```python
from build123d import *

# Parameters (mm, degrees)
SKETCH1_W               = 56
SKETCH1_H               = 32
BOSS_EXTRUDE1_DEPTH     = 2
SKETCH2_R               = 1.75
CUT_EXTRUDE1_DEPTH      = 33.310988843
MIRROR2_COPY_1_SKETCH_R = 1.75
MIRROR2_COPY_1_DEPTH    = 33.310988843
SKETCH4_W               = 14.25
SKETCH4_H               = 7.5
CUT_EXTRUDE2_DEPTH      = 33.310988843
MIRROR4_COPY_1_SKETCH_W = 14.25
MIRROR4_COPY_1_SKETCH_H = 7.5
MIRROR4_COPY_1_DEPTH    = 33.310988843
SKETCH5_W               = 56
SKETCH5_H               = 32
SKETCH5_W_2             = 50
SKETCH5_H_2             = 26
BOSS_EXTRUDE2_DEPTH     = 4.65
SKETCH6_W               = 51
SKETCH6_H               = 27
SKETCH6_W_2             = 50
SKETCH6_H_2             = 26
BOSS_EXTRUDE3_DEPTH     = 1
FILLET1_R               = 1


with BuildPart() as part:
    # Sketch1 → Boss-Extrude1 (new body)
    with BuildSketch(Plane(origin=(0, 0, 0), x_dir=(1, 0, 0), z_dir=(0, 1, 0))):
        Rectangle(SKETCH1_W, SKETCH1_H)
    extrude(amount=BOSS_EXTRUDE1_DEPTH)

    # Sketch2 → Cut-Extrude1 (cut, through all)
    with BuildSketch(Plane(origin=(0, 0, 0), x_dir=(1, 0, 0), z_dir=(0, 1, 0))):
        with Locations(Location((20, 6.5, 0), (0, 0, 270))):
            Circle(SKETCH2_R)
    cut_extrude1 = extrude(amount=CUT_EXTRUDE1_DEPTH, mode=Mode.SUBTRACT)

    # Mirror1: Cut-Extrude1 across plane
    add(cut_extrude1.mirror(Plane.XY), mode=Mode.SUBTRACT)

    # Mirror2: Cut-Extrude1 across plane
    add(cut_extrude1.mirror(Plane(origin=(0, 0, 0), x_dir=(0, 0, 1), z_dir=(1, 0, 0))), mode=Mode.SUBTRACT)

    # Mirror2 copy 1 sketch → Mirror2 copy 1 (cut, through all)
    with BuildSketch(Plane(origin=(0, 0, 0), x_dir=(-1, 0, 0), z_dir=(0, 1, 0))):
        with Locations(Location((20, 6.5, 0), (0, 0, 270))):
            Circle(MIRROR2_COPY_1_SKETCH_R)
    extrude(amount=MIRROR2_COPY_1_DEPTH, mode=Mode.SUBTRACT)

    # Sketch4 → Cut-Extrude2 (cut, through all)
    with BuildSketch(Plane(origin=(0, 0, 0), x_dir=(1, 0, 0), z_dir=(0, 1, 0))):
        with Locations((8.46, 6.875)):
            Rectangle(SKETCH4_W, SKETCH4_H)
    cut_extrude2 = extrude(amount=CUT_EXTRUDE2_DEPTH, mode=Mode.SUBTRACT)

    # Mirror3: Cut-Extrude2 across plane
    add(cut_extrude2.mirror(Plane(origin=(0, 0, 0), x_dir=(0, 0, 1), z_dir=(1, 0, 0))), mode=Mode.SUBTRACT)

    # Mirror4: Cut-Extrude2 across plane
    add(cut_extrude2.mirror(Plane.XY), mode=Mode.SUBTRACT)

    # Mirror4 copy 1 sketch → Mirror4 copy 1 (cut, through all)
    with BuildSketch(Plane(origin=(0, 0, 0), x_dir=(-1, 0, 0), z_dir=(0, 1, 0))):
        with Locations((8.46, 6.875)):
            Rectangle(MIRROR4_COPY_1_SKETCH_W, MIRROR4_COPY_1_SKETCH_H)
    extrude(amount=MIRROR4_COPY_1_DEPTH, mode=Mode.SUBTRACT)

    # Sketch5 → Boss-Extrude2 (add)
    with BuildSketch(Plane.XZ):
        Rectangle(SKETCH5_W, SKETCH5_H)
        Rectangle(SKETCH5_W_2, SKETCH5_H_2, mode=Mode.SUBTRACT)
    extrude(amount=BOSS_EXTRUDE2_DEPTH)

    # Sketch6 → Boss-Extrude3 (add)
    with BuildSketch(Plane.XZ.offset(4.65)):
        Rectangle(SKETCH6_W, SKETCH6_H)
        Rectangle(SKETCH6_W_2, SKETCH6_H_2, mode=Mode.SUBTRACT)
    extrude(amount=BOSS_EXTRUDE3_DEPTH)

    # Fillet1
    fillet1_edges = [part.edges().sort_by_distance(p)[0] for p in [
        (-25.5, -5.15, -13.5),
        (25.5, -5.15, -13.5),
        (25.5, -5.15, 13.5),
        (-25.5, -5.15, 13.5),
        (28, -1.325, 16),
        (-28, -1.325, 16),
        (-28, -1.325, -16),
        (28, -1.325, -16),
        (25, -2.825, -13),
        (25, -2.825, 13),
        (-25, -2.825, 13),
        (-25, -2.825, -13),
    ]]
    fillet(fillet1_edges, radius=FILLET1_R)


solid = part.part
```
CAD build for the part. Positions are in the model's coordinates, mm. A direction names the side the tool comes from. Round coordinates to 2 decimals unless told otherwise and drop trailing zeros. Order: outer loops, then holes, each group sorted by start corner. A loop starts at its lowest first (then second) coordinate and runs counter-clockwise, first axis right, second up.
Item 1: Saw through at A-A on x = -20. Write the cut outline in (y, z), then the cut area to 3 significant figures.
Item 2: Saw through at C-C on y = -3.25. Write the cut outline in (x, z), then the cut area to 3 significant figures.
Item 3: Saw through at B-B on z = -6.5. Write the cut outline in (x, y) (3 decimals).
Item 4: Probe line 1 along Z through (x, y) = (-20, 0.5); line 2 along X through (y, z) = (1.4, 6.5) (3 decimals); line 3 along Z through (x, y) = (-11, 1.25) (3 decimals). List the from-to ranges inside material, lowest first.
Item 5: Mould opens along Z. For faces 1 (the face through (-27.699, -1.372, -15.715)), 2 (the face through (-28, -1, 0)), 3 (the face through (-15.585, 1, -7)) say: pulls with the +Z half, pulls with the -Z half, needs draft (parallel to the pull), parting line crosses it, or undercut.
Item 6: Saw through at D-D on x = 17.5. Write the cut outline in (y, z), then the cut area to 3 significant figures.
Item 7: Tool access for faces 4 (the face through (-1.335, 1, -7)), 5 (the face through (0, -5, 13.5)), 6 (the face through (24.715, -2.785, -12.699)): list every direction of +Z, -Z, +X, -X, +Y, -Y with a clear straight run to the whole face (end or side of a thin tool).
Reported:
1. outline: (-5.65, -13.5) - (-4.65, -13.5) - (-4.65, -16) - (2, -16) - (2, -8.25) - (0, -8.25) - (0, -13) - (-5.65, -13) - close; (-5.65, 13) - (0, 13) - (0, 8.25) - (2, 8.25) - (2, 16) - (-4.65, 16) - (-4.65, 13.5) - (-5.65, 13.5) - close; (0, -4.75) - (2, -4.75) - (2, 4.75) - (0, 4.75) - close
1. area: 78.9 mm2
2. outline: (-28, -15) arc R1 ccw to (-27, -16) - (27, -16) arc R1 ccw to (28, -15) - (28, 15) arc R1 ccw to (27, 16) - (-27, 16) arc R1 ccw to (-28, 15) - close; hole (-25, -12) arc R1 ccw to (-24, -13) - (24, -13) arc R1 ccw to (25, -12) - (25, 12) arc R1 ccw to (24, 13) - (-24, 13) arc R1 ccw to (-25, 12) - close
2. area: 492 mm2
3. outline: (-28, -4.65) - (-25.5, -4.65) - (-25.5, -5.65) - (-25, -5.65) - (-25, 0) - (-21.75, 0) - (-21.75, 2) - (-28, 2) - close; (-18.25, 0) - (-15.585, 0) - (-15.585, 2) - (-18.25, 2) - close; (-1.335, 0) - (1.335, 0) - (1.335, 2) - (-1.335, 2) - close; (15.585, 0) - (18.25, 0) - (18.25, 2) - (15.585, 2) - close; (21.75, 0) - (25, 0) - (25, -5.65) - (25.5, -5.65) - (25.5, -4.65) - (28, -4.65) - (28, 2) - (21.75, 2) - close
4. line 1: z = -16 to -8.25, -4.75 to 4.75, 8.25 to 16
4. line 2: x = -28 to -21.75, -18.25 to -15.585, -1.335 to 1.335, 15.585 to 18.25, 21.75 to 28
4. line 3: z = -16 to -10.625, -3.125 to 3.125, 10.625 to 16
5. face 1: pulls with the -Z half
5. face 2: needs draft
5. face 3: undercut
6. outline: (-5.65, -13.5) - (-4.65, -13.5) - (-4.65, -16) - (2, -16) - (2, 16) - (-4.65, 16) - (-4.65, 13.5) - (-5.65, 13.5) - (-5.65, 13) - (0, 13) - (0, -13) - (-5.65, -13) - close
6. area: 92.9 mm2
7. face 4: +Y, -Y
7. face 5: +Z, +X, -X, -Y
7. face 6: -Y
